from build123d import *
from build123d.topology import SkipClean

# Parameters (mm, degrees)
SKETCH_1_R          = 37.5
SKETCH_1_R_2        = 29
EXTRUDE_1_DEPTH     = 4
SKETCH_2_R          = 37.5
SKETCH_2_R_2        = 36
EXTRUDE_2_DEPTH     = 5
EXTRUDE_START       = 84.5
SKETCH_3_R          = 37.5
SKETCH_3_R_2        = 29
EXTRUDE_3_DEPTH     = 84.5
SKETCH_4_W          = 100
SKETCH_4_H          = 80
SKETCH_4_R          = 37.5
EXTRUDE_4_DEPTH     = 3
SKETCH_5_R          = 5
SKETCH_5_R_2        = 2.15
EXTRUDE_5_DEPTH     = 93.5
EXTRUDE_5_2_DEPTH   = 93.5
EXTRUDE_START_2     = -3
EXTRUDE_6_DEPTH     = 93.5
SKETCH_8_R          = 35
CUT_EXTRUDE_1_DEPTH = 87.5
CHAMFER_1_SIZE      = 6
CUT_EXTRUDE_2_DEPTH = 116.509739972


with BuildPart() as part:
    # 草图1 → 凸台-拉伸1 (new body)
    with BuildSketch(Plane(origin=(0, 0, 0), x_dir=(1, 0, 0), z_dir=(0, 1, 0))):
        with Locations(Location((0, 0, 0), (0, 0, 270))):
            Circle(SKETCH_1_R)
        with Locations(Location((0, 0, 0), (0, 0, 270))):
            Circle(SKETCH_1_R_2, mode=Mode.SUBTRACT)
    extrude(amount=EXTRUDE_1_DEPTH)

    # 草图2 → 凸台-拉伸2 (add)
    with BuildSketch(Plane(origin=(0, 4, 0), x_dir=(1, 0, 0), z_dir=(0, 1, 0))):
        with Locations(Location((0, 0, 0), (0, 0, 270))):
            Circle(SKETCH_2_R)
        with Locations(Location((0, 0, 0), (0, 0, 270))):
            Circle(SKETCH_2_R_2, mode=Mode.SUBTRACT)
    extrude(amount=EXTRUDE_2_DEPTH)

    # 草图3 → 凸台-拉伸3 (add)
    with BuildSketch(Plane.XZ.offset(EXTRUDE_START)):
        with Locations(Location((0, 0, 0), (0, 0, 270))):
            Circle(SKETCH_3_R)
        with Locations(Location((0, 0, 0), (0, 0, 270))):
            Circle(SKETCH_3_R_2, mode=Mode.SUBTRACT)
    extrude(amount=-EXTRUDE_3_DEPTH)

    # 草图4 → 凸台-拉伸4 (add)
    with BuildSketch(Plane.XZ.offset(84.5)):
        Rectangle(SKETCH_4_W, SKETCH_4_H)
        with Locations(Location((0, 0, 0), (0, 0, 270))):
            Circle(SKETCH_4_R, mode=Mode.SUBTRACT)
    extrude(amount=-EXTRUDE_4_DEPTH)

    # 草图6 → 凸台-拉伸6 (add)
    with SkipClean():  # the faces are left unmerged after this step: merging them gives an invalid solid
        with BuildSketch(Plane(origin=(0, -81.5, 0), x_dir=(1, 0, 0), z_dir=(0, 1, 0)).offset(EXTRUDE_START_2)):
            with BuildLine():
                Line((-4.698463104, 48.210100717), (-8.995097405, 36.405194996))
                ThreePointArc((-8.995097405, 36.405194996), (0, 37.5), (8.995097405, 36.405194996))
                Line((8.995097405, 36.405194996), (4.698463104, 48.210100717))
                ThreePointArc((4.698463104, 48.210100717), (0, 41.5), (-4.698463104, 48.210100717))
            make_face()
            with BuildLine():
                Line((4.698463104, -48.210100717), (8.995097405, -36.405194996))
                ThreePointArc((8.995097405, -36.405194996), (0, -37.5), (-8.995097405, -36.405194996))
                Line((-8.995097405, -36.405194996), (-4.698463104, -48.210100717))
                ThreePointArc((-4.698463104, -48.210100717), (0, -41.5), (4.698463104, -48.210100717))
            make_face()
        extrude(amount=EXTRUDE_6_DEPTH)


with BuildPart() as body_2:
    # 草图5 → 凸台-拉伸5 (new body)
    with BuildSketch(Plane.XZ.offset(84.5)):
        with Locations(Location((0, 46.5, 0), (0, 0, 270))):
            Circle(SKETCH_5_R)
        with Locations(Location((0, 46.5, 0), (0, 0, 270))):
            Circle(SKETCH_5_R_2, mode=Mode.SUBTRACT)
    extrude(amount=-EXTRUDE_5_DEPTH)


with BuildPart() as body_3:
    # 草图5 → Extrude 5 2 (new body)
    with BuildSketch(Plane.XZ.offset(84.5)):
        with Locations(Location((0, -46.5, 0), (0, 0, 270))):
            Circle(SKETCH_5_R)
        with Locations(Location((0, -46.5, 0), (0, 0, 270))):
            Circle(SKETCH_5_R_2, mode=Mode.SUBTRACT)
    extrude(amount=-EXTRUDE_5_2_DEPTH)

    # Combine 2: union body 2, part
    add(body_2.part)
    add(part.part)

    # 草图8 → 切除-拉伸1 (cut)
    with BuildSketch(Plane.XZ.offset(84.5)):
        with Locations(Location((0, 0, 0), (0, 0, 270))):
            Circle(SKETCH_8_R)
    extrude(amount=-CUT_EXTRUDE_1_DEPTH, mode=Mode.SUBTRACT)

    # 倒角1
    chamfer_1_edges = [body_3.edges().sort_by_distance(p)[0] for p in [
        (0, 3, 35),
    ]]
    chamfer(chamfer_1_edges, length=CHAMFER_1_SIZE - 0.0001)  # a hair under: the kernel refuses the full size

    # 草图9 → 切除-旋转1 (revolve, cut)
    with BuildSketch(Plane.XY, mode=Mode.PRIVATE) as cut_revolve_1_sk:
        Polygon((-37.5, -9), (-60, 13.5), (-60, -74.5), (-37.5, -74.5), align=None)
    revolve(cut_revolve_1_sk.sketch.rotate(Axis((0, 9, 0), (0, -1, 0)), 76.121175643), axis=Axis((0, 9, 0), (0, -1, 0)), mode=Mode.SUBTRACT)

    # 草图11 → 切除-拉伸2 (cut, through all)
    with BuildSketch(Plane(origin=(0, -81.5, 0), x_dir=(1, 0, 0), z_dir=(0, 1, 0))):
        with BuildLine():
            Line((-20.615528128, 40), (-50, 40))
            Line((-50, 40), (-50, -40))
            Line((-50, -40), (-20.615528128, -40))
            ThreePointArc((-20.615528128, -40), (-45, 0), (-20.615528128, 40))
        make_face()
        with BuildLine():
            Line((20.615528128, 40), (50, 40))
            Line((50, 40), (50, -40))
            Line((50, -40), (20.615528128, -40))
            ThreePointArc((20.615528128, -40), (45, 0), (20.615528128, 40))
        make_face()
    extrude(amount=-CUT_EXTRUDE_2_DEPTH, mode=Mode.SUBTRACT)


solid = body_3.part
Can you work these out from the model? Positions are in its coordinate system, mm. A direction names the side the tool comes from. Give positions to 0.01 mm unless a question says otherwise; leave off trailing zeros. Write each loop counter-clockwise with the first axis right and the second up, starting at its lowest first coordinate (ties: lowest second). Pieces come first, ordered by that corner, then holes. Notation, with made-up numbers: (-14.5, 16.25) -> (-1.5, 16.25) arc R27 cw to (-1.5, 40.25) -> close; hole circle Ø4 at (-28, 87.25). An arc over 180 degrees is marked (long way). Answer as a JSON object with one key per item and string values. Group by question number.
Item 1: I'm going to push flat-ended pins straight in: P1, Ø2.5, axis at x = 0, z = 46.5, coming from the -Y side; P2, Ø0.9, axis at x = 13.5, y = -83.5, coming from the -Z side; P3, Ø4, axis at y = -68, z = -3, coming from the -X side; P4, Ø1.5, axis at x = 13, y = -83.5, coming from the +Z side. Where does each tip first touch, or does it pass through?
Item 2: Suppose I cut it at B-B (y = -38). Please give me the cut outline in (x, z).
Item 3: We'd pull the mould along Z, two halves only. Please class faces 6 (the face through (-14, -83, 40)), 7 (the face through (10.81, 6.46, 34.34)), 8 (the face through (1, -74.5, -43)), 9 (the face through (7.354, 1.874, -40.913)): +Z half, -Z half, draft (parallel to the pull), parting line (faces both ways), or undercut.
Item 4: Suppose I cut it at C-C (x = 0). State how many separate pieces and enclosed holes the cut face has, plus the area to 3 significant figures.
Item 5: Please list where these lines run through material, in increasing order: line 1 (X direction, y = -74, z = -0.5); line 2 (X direction, y = 3, z = 0); line 3 (Z direction, x = 0, y = 3). Write a range as [from, to].
Item 6: For faces 1 (the face through (-14, -83, -40)), 2 (the face through (14, -83, -40)), 3 (the face through (-21, -44, 28)), 4 (the face through (39, -81.5, 0)), 5 (the face through (14, -83, 40)), which set-ups out of +Z, -Z, +X, -X, +Y, -Y let a thin tool reach every point of the face, with its end or its side?
Findings:
{
 "1": {"P1": "passes through", "P2": "stops at z = -40", "P3": "stops at x = -37.49", "P4": "stops at z = 40"},
 "2": {"outline": "circle Ø75 at (0, 0); hole circle Ø70 at (0, 0)"},
 "3": {"face 6": "+Z half", "face 7": "undercut", "face 8": "draft", "face 9": "-Z half"},
 "4": {"separate pieces": "6", "enclosed holes": "0", "area": "930 mm²"},
 "5": {"line 1": "x = [-37.5, -35], [35, 37.5]", "line 2": "x = [-37.5, -29], [29, 37.5]", "line 3": "z = [-49.5, -48.65], [-44.35, -29], [29, 44.35], [48.65, 49.5]"},
 "6": {"face 1": "-Z, -X, +Y, -Y", "face 2": "-Z, +X, +Y, -Y", "face 3": "-Y", "face 4": "+X, +Y", "face 5": "+Z, +X, +Y, -Y"}
}
